```python
from build123d import *

# Parameters (mm, degrees)
F0_W      = 334.6
F0_H      = 73.025
F1_DEPTH  = 25.4
F2_SIZE   = 5.08
F4_D      = 6.8
F4_DEPTH  = 23.15
F4_TIP    = 2.0429261047
F6_D      = 6.8
F6_DEPTH  = 23.1394
F6_TIP    = 2.0429261047
F8_D      = 6.6
F10_DEPTH = 25.4
F12_DEPTH = 25.4


# Not quite as in the source:
# - a feature names something its author has since deleted; it is built from what else it names


with BuildPart() as f1:
    # F0 (on Top) → F1 (new body)
    with BuildSketch(Plane.XY):
        with Locations((164.5870582715, 36.5125)):
            Rectangle(F0_W, F0_H)
    extrude(amount=F1_DEPTH)

    # F2
    f2_edges = [f1.edges().sort_by_distance(p)[0] for p in [
        (164.587058, 73.025, 25.4),
    ]]
    chamfer(f2_edges, length=F2_SIZE)

    # F4
    with Locations(Plane.YZ.offset(331.8870582715)):
        with Locations((34.925, 12.7), (60.325, 12.7)):
            Hole(F4_D / 2, depth=F4_DEPTH)
            with Locations((0, 0, -(F4_DEPTH + F4_TIP / 2))):  # 118° drill point
                Cone(0, F4_D / 2, F4_TIP, mode=Mode.SUBTRACT)

    # F6
    with Locations(Plane(origin=(-2.7129417285, 0, 0), x_dir=(0, -1, 0), z_dir=(-1, 0, 0))):
        with Locations((-60.325, 12.7), (-34.925, 12.7)):
            Hole(F6_D / 2, depth=F6_DEPTH)
            with Locations((0, 0, -(F6_DEPTH + F6_TIP / 2))):  # 118° drill point
                Cone(0, F6_D / 2, F6_TIP, mode=Mode.SUBTRACT)

    # F8 (through all)
    with Locations(Plane.XY.offset(25.4)):
        with Locations((289.6185582715, 8.89), (289.6185582715, 59.055)):
            Hole(F8_D / 2)

    # F9 (on face) → F10 (cut)
    with BuildSketch(Plane.XY.offset(25.4)):
        with BuildLine():
            ThreePointArc((286.3185582715, 8.89), (289.6185582715, 12.19), (292.9185582715, 8.89))
            Line((292.9185582715, 8.89), (292.9185582715, 59.055))
            ThreePointArc((292.9185582715, 59.055), (289.6185582715, 55.755), (286.3185582715, 59.055))
            Line((286.3185582715, 59.055), (286.3185582715, 8.89))
        make_face()
    extrude(amount=-F10_DEPTH, mode=Mode.SUBTRACT)

    # F11 (on face) → F12 (cut)
    with BuildSketch(Plane.XY.offset(25.4)):
        with BuildLine():
            ThreePointArc((236.3059582715, 8.89), (239.6059582715, 5.59), (242.9059582715, 8.89))
            Line((242.9059582715, 8.89), (242.9059582715, 59.055))
            ThreePointArc((242.9059582715, 59.055), (239.6059582715, 62.355), (236.3059582715, 59.055))
            Line((236.3059582715, 59.055), (236.3059582715, 8.89))
        make_face()
        with BuildLine():
            ThreePointArc((186.2933582715, 8.89), (189.5933582715, 5.59), (192.8933582715, 8.89))
            Line((192.8933582715, 8.89), (192.8933582715, 59.055))
            ThreePointArc((192.8933582715, 59.055), (189.5933582715, 62.355), (186.2933582715, 59.055))
            Line((186.2933582715, 59.055), (186.2933582715, 8.89))
        make_face()
        with BuildLine():
            ThreePointArc((136.2807582715, 8.89), (139.5807582715, 5.59), (142.8807582715, 8.89))
            Line((142.8807582715, 8.89), (142.8807582715, 59.055))
            ThreePointArc((142.8807582715, 59.055), (139.5807582715, 62.355), (136.2807582715, 59.055))
            Line((136.2807582715, 59.055), (136.2807582715, 8.89))
        make_face()
        with BuildLine():
            ThreePointArc((86.2681582715, 8.89), (89.5681582715, 5.59), (92.8681582715, 8.89))
            Line((92.8681582715, 8.89), (92.8681582715, 59.055))
            ThreePointArc((92.8681582715, 59.055), (89.5681582715, 62.355), (86.2681582715, 59.055))
            Line((86.2681582715, 59.055), (86.2681582715, 8.89))
        make_face()
        with BuildLine():
            ThreePointArc((36.2555582715, 8.89), (39.5555582715, 5.59), (42.8555582715, 8.89))
            Line((42.8555582715, 8.89), (42.8555582715, 59.055))
            ThreePointArc((42.8555582715, 59.055), (39.5555582715, 62.355), (36.2555582715, 59.055))
            Line((36.2555582715, 59.055), (36.2555582715, 8.89))
        make_face()
    extrude(amount=-F12_DEPTH, mode=Mode.SUBTRACT)


solid = f1.part
```
Model file for the job. Use its own axes, mm. A direction names the side the tool comes from. Round coordinates to 2 decimals unless told otherwise and drop trailing zeros. Order: outer loops, then holes, each group sorted by start corner. A loop starts at its lowest first (then second) coordinate and runs counter-clockwise, first axis right, second up. Notation, with made-up numbers: (-31.5, 44.5) -> (-7.5, 44.5) arc R20 ccw to (-7.5, 68.5) -> close; hole circle Ø4 at (87, 30.5). An arc over 180 degrees is marked (long way). Use one line per item in the form item = value.
Item 1: Cut at A-A, the plane y = 49. Write the cut outline in (x, z).
Returned:
outline = (-2.71, 0) -> (36.26, 0) -> (36.26, 25.4) -> (-2.71, 25.4) -> close; (42.86, 0) -> (86.27, 0) -> (86.27, 25.4) -> (42.86, 25.4) -> close; (92.87, 0) -> (136.28, 0) -> (136.28, 25.4) -> (92.87, 25.4) -> close; (142.88, 0) -> (186.29, 0) -> (186.29, 25.4) -> (142.88, 25.4) -> close; (192.89, 0) -> (236.31, 0) -> (236.31, 25.4) -> (192.89, 25.4) -> close; (242.91, 0) -> (286.32, 0) -> (286.32, 25.4) -> (242.91, 25.4) -> close; (292.92, 0) -> (331.89, 0) -> (331.89, 25.4) -> (292.92, 25.4) -> close
Item 2: Pull direction Y, two halves, no side cores. Call faces 4 (the face through (162, 73.025, 10)), 5 (the face through (22.115, 60.008, 13.198)), 6 (the face through (239.679, 62.354, 12.878)), 7 (the face through (331.887, 36, 18)): released by +Y, released by -Y, zero draft, split by the parting line, or undercut.
Returned:
face_4 = released by +Y
face_5 = undercut
face_6 = undercut
face_7 = zero draft
Item 3: Flat gauge pins, fed straight in: pin 1 Ø11 at (y, z) = (60.325, 12.7) entering from -X; pin 2 Ø6 at (y, z) = (60.325, 12.7) entering from -X. Where does each tip first touch, or does it go through?
Returned:
pin_1 = -2.71
pin_2 = 20.67
Item 4: Tool access for faces 1 (the face through (186.293, 34, 13)), 2 (the face through (9.02, 56.93, 12.85)), 3 (the face through (320.15, 38.32, 12.85)): list every direction of +Z, -Z, +X, -X, +Y, -Y with a clear straight run to the whole face (end or side of a thin tool).
Returned:
face_1 = +Z, -Z
face_2 = -X
face_3 = +X
Item 5: Drill centre lines: line 1 (Y direction, x = 325, z = 12.7) (3 decimals); line 2 (Y direction, x = 140, z = 24.25) (3 decimals); line 3 (Z direction, x = 225, y = 69) (3 decimals). Where is each one in solid material? Low to high.
Returned:
line_1 = 0 to 31.525, 38.325 to 56.925, 63.725 to 73.025
line_2 = 0 to 5.617, 62.328 to 69.095
line_3 = 0 to 24.345
